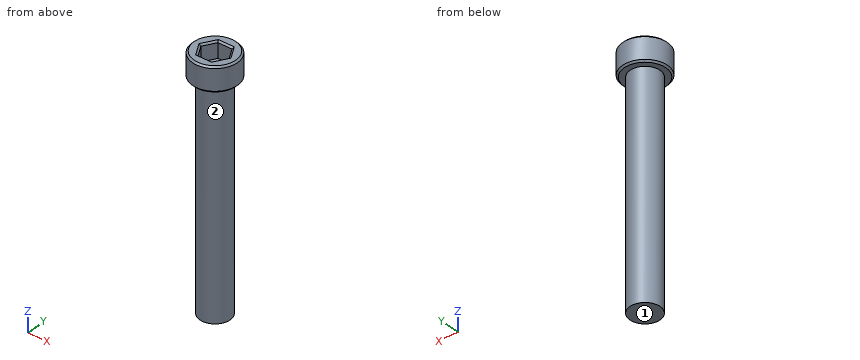
Autodesk Inventor part; units mm, degrees
ref_plane "YZ Plane" through (0, 0, 0) normal (1, 0, 0) x (0, 1, 0)
ref_plane "XZ Plane" through (0, 0, 0) normal (0, 1, 0) x (-1, 0, 0)
ref_plane "XY Plane" through (0, 0, 0) normal (0, 0, 1) x (1, 0, 0)
sketch "Sketch1" plane through (0, 0, 0) normal (0, 0, 1) x (1, 0, 0)
  circle A0 centre (0, 0) radius 3.4925
  circle A1 centre (0, 0) radius 2.3495
  line L0 (2.1997, 0) -> (1.0999, -1.905)
  line L1 (1.0999, -1.905) -> (-1.0999, -1.905)
  line L2 (-1.0999, -1.905) -> (-2.1997, 0)
  line L3 (-2.1997, 0) -> (-1.0999, 1.905)
  line L4 (-1.0999, 1.905) -> (1.0999, 1.905)
  line L5 (1.0999, 1.905) -> (2.1997, 0)
  dimension "d0" = 6.985
  dimension "d1" = 4.699
  dimension "d2" = 3.81
extrude "Extrusion1" add sketch "Sketch1" along normal blind 3.81 contours A0 | A1
extrude "Extrusion2" add sketch "Sketch1" against normal blind 34.29 contours A1 | L0 L1 L2 L3 L4 L5
extrude "Extrusion3" add sketch "Sketch1" along normal blind 1.27 contours L0 L1 L2 L3 L4 L5
thread "Thread1"
chamfer "Chamfer1" distance 0.254 angle 45 8 edges at (-3.4925, 0, 3.81) (-3.4925, 0, 0) (-1.6498, 0.9525, 3.81) (-1.6498, -0.9525, 3.81) (0, -1.905, 3.81) (1.6498, -0.9525, 3.81) (1.6498, 0.9525, 3.81) (0, 1.905, 3.81)
properties part number "Gearbox Hex Machine Screw 2" material "Steel"
Can you work these out from the model? Positions are in its coordinate system, mm. Face numbers are marked on the shaded views. A direction names the side the tool comes from. Coordinates: 2 decimals unless noted, no trailing zeros. Loops run counter-clockwise (first coordinate to the right, second up) from the corner with the lowest first, then second, coordinate; pieces in that order, holes last. Notation, with made-up numbers: (14, 16) - (62, 16) arc R15 cw to (62, 20) - close; hole circle Ø2 at (-23.75, 34). An arc over 180 degrees is marked (long way). Answer as CSV lines item,"result". Start each with the question number.
1) I need wall thicknesses on line 1 (Z direction, x = -1.25, y = -0.75); line 2 (Z direction, x = 0.75, y = 3); line 3 (Y direction, x = 2, z = -24.5). Which ranges of each line are inside material? Lowest first, please. Write a range as from..to.
2) Which directions (+Z, -Z, +X, -X, +Y, -Y) give clear straight access to the entire face, cutting with the end or side of a thin tool? Please do the marked faces 1 and 2.
3) Suppose I cut it at B-B (z = -17.5). Please give me the cut outline in (x, y), plus the area to 3 significant figures.
4) For pin 1 (1.1 mm diameter, centred on x = -0.5, y = -1, fed in from +Z); pin 2 (1.5 mm diameter, centred on y = -2.5, z = -17, fed in from -X); pin 3 (0.7 mm diameter, centred on x = 0.5, z = 3, fed in from +Y), each with a flat end and sliding along its axis, tell me the tip position at first contact or that it passes through.
Check result:
1,line 1,"z = -34.29..1.27"
1,line 2,"z = 0..3.81"
1,line 3,"y = -1.23..1.23"
2,face 1,"-Z, +X, -X, +Y, -Y"
2,face 2,"-Z"
3,outline,"circle Ø4.7 at (0, 0)"
3,area,"17.3 mm²"
4,pin 1,"stops at z = 1.27"
4,pin 2,"stops at x = -1.57"
4,pin 3,"stops at y = 3.49"
